from build123d import *

# Parameters (mm, degrees)
SKETCH1_R           = 31.65
BOSS_EXTRUDE1_DEPTH = 11
CUT_EXTRUDE1_DEPTH  = 35.5
SKETCH3_R           = 3.375
CUT_EXTRUDE2_DEPTH  = 21
SKETCH4_R           = 14.25
BOSS_EXTRUDE2_DEPTH = 62
SHELL1_T            = -4.2


# Read off the part's stored shape, not the designer's step: Draft1, Split1
with BuildPart() as part:
    # Sketch1 → Boss-Extrude1 (new body)
    with BuildSketch(Plane(origin=(0, 0, 0), x_dir=(1, 0, 0), z_dir=(0, 1, 0))):
        with Locations(Location((0, 0, 0), (0, 0, 270))):
            Circle(SKETCH1_R)
    extrude(amount=BOSS_EXTRUDE1_DEPTH)

    # Sketch2 → Cut-Extrude1 (cut, symmetric)
    with BuildSketch(Plane(origin=(0, 0, 0), x_dir=(0, 0, -1), z_dir=(1, 0, 0))):
        Polygon((31.65, 11), (-31.65, 4.5), (-31.65, 11), align=None)
    extrude(amount=CUT_EXTRUDE1_DEPTH, both=True, mode=Mode.SUBTRACT)

    # Sketch3 → Cut-Extrude2 (cut)
    with BuildSketch(Plane(origin=(0, 7.669134063, 0.787509817), x_dir=(1, 0, 0), z_dir=(0, 0.9947691619431022, 0.10214849214265666))):
        with Locations(Location((0, -25.899775761, 0), (0, 0, 270))):
            Circle(SKETCH3_R)
        with Locations(Location((-22.429863761, -12.94988788, 0), (0, 0, 270))):
            Circle(SKETCH3_R)
        with Locations(Location((-22.429863761, 12.94988788, 0), (0, 0, 270))):
            Circle(SKETCH3_R)
        with Locations(Location((0, 25.899775761, 0), (0, 0, 270))):
            Circle(SKETCH3_R)
        with Locations(Location((22.429863761, 12.94988788, 0), (0, 0, 270))):
            Circle(SKETCH3_R)
        with Locations(Location((22.429863761, -12.94988788, 0), (0, 0, 270))):
            Circle(SKETCH3_R)
    extrude(amount=-CUT_EXTRUDE2_DEPTH, mode=Mode.SUBTRACT)

    # Sketch4 → Boss-Extrude2 (add)
    with BuildSketch(Plane(origin=(0, 7.669134063, 0.787509817), x_dir=(1, 0, 0), z_dir=(0, 0.9947691619431022, 0.10214849214265666))):
        with Locations(Location((0, 0.791650814, 0), (0, 0, 270))):
            Circle(SKETCH4_R)
    extrude(amount=-BOSS_EXTRUDE2_DEPTH)

    # Draft1 outline → Draft1 (revolve)
    with BuildSketch(Plane(origin=(0, 0.080865937, -0.787509817), x_dir=(1, 0, 0), z_dir=(0, -0.102148492142657, 0.994769161943102))):
        Polygon((14.25, -54.290538995), (17.183507111, 1.684111168), (14.25, 1.684111168), align=None)
    revolve(axis=Axis((0, 0.080865937, -0.787509817), (0, 0.994769161943102, 0.102148492142657)))


with BuildPart() as body_2:
    # Split1: the piece on the far side of the plane
    add(part.part)
    split(bisect_by=Plane(origin=(0, 0, 0), x_dir=(1, 0, 0), z_dir=(0, 1, 0)), keep=Keep.BOTTOM)

    # Shell1
    shell1_openings = [body_2.faces().sort_by_distance(p)[0] for p in [
        (0, -53.92568804, -6.333206513),
    ]]
    offset(amount=SHELL1_T, openings=shell1_openings, kind=Kind.INTERSECTION)


with BuildPart() as part_1:
    add(part.part)

    # Split1
    split(bisect_by=Plane(origin=(0, 0, 0), x_dir=(1, 0, 0), z_dir=(0, 1, 0)), keep=Keep.TOP)


with BuildPart() as body_2_1:
    add(body_2.part)

    # Combine1: union part
    add(part_1.part)


solid = body_2_1.part
CAD build for the part. Positions are in the model's coordinates, mm. A direction names the side the tool comes from. Give positions to 0.01 mm unless a question says otherwise; leave off trailing zeros. Write each loop counter-clockwise with the first axis right and the second up, starting at its lowest first coordinate (ties: lowest second). Pieces come first, ordered by that corner, then holes. Notation, with made-up numbers: M 21.5,53 L 78.5,53 A28 ccw 78.5,83 Z; hole C -7.75,34 d6. An arc over 180 degrees is marked long. Put each result on its own line as item: value. Start each with the question number.
(1) Flat gauge pins, fed straight in: pin 1 Ø10 at (y, z) = (-18, 5) entering from -X; pin 2 Ø7.5 at (x, z) = (-4, -6) entering from -Y; pin 3 Ø3 at (x, z) = (-9, -4.5) entering from -Y. Where does each tip first touch, or does it go through?
(2) Mould opens along Y. For faces 3 (the face through (22.578, 4.717, -15.923)), 4 (the face through (-2.473, -29.177, 7.403)), 5 (the face through (0.443, 7.795, -0.443)) say: +Y half, -Y half, draft (parallel to the pull), parting line (faces both ways), or undercut.
(3) Band-saw the part on B-B, the plane z = -12. Give the number of separate pieces and of enclosed holes in the cut face, and give its area (3 significant figures).
(4) Band-saw the part on A-A, the plane x = -21. Write the cut outline in (y, z), and give its area (3 significant figures).
(5) Which spindle directions (+Z, -Z, +X, -X, +Y, -Y) get a long thin tool onto all of the face, cutting with end or side? Do faces 1 (the face through (9.699, -53.582, -9.682)), 2 (the face through (0, -4.2, -1)). Say none if no direction does.
(6) Probe L1, parallel to X at y = -32, z = -4.5; L2, parallel to Z at x = -9, y = -35; L3, parallel to X at y = -32, z = 5.5. List the from-to ranges inside material, lowest first.
(7) Band-saw the part on C-C, the plane x = 0. Write the cut outline in (y, z).
Response values:
1. pin 1: stops at x = -16.01
1. pin 2: stops at y = -4.2
1. pin 3: stops at y = -54.26
2. face 3: parting line
2. face 4: undercut
2. face 5: +Y half
3. separate pieces: 3
3. enclosed holes: 0
3. area: 1,050 mm2
4. outline: M 0,-23.68 L 10.18,-23.68 L 9.3,-15.14 L 0,-16.09 Z; M 0,-9.94 L 8.68,-9.05 L 6.66,10.63 L 0,9.94 Z; M 0,16.09 L 6.03,16.71 L 5.32,23.68 L 0,23.68 Z
4. area: 273 mm2
5. face 1: -Z, +X, -X, -Y
5. face 2: none
6. L1: x = -15.4 to -11.19, 11.19 to 15.4
6. L2: z = -16.68 to -10.76, 2.1 to 8.07
6. L3: x = -12.17 to -5.98, 5.98 to 12.17
7. outline: M -55.38,7.84 L -54.95,3.66 L -4.2,11.57 L -4.2,-13.89 L -52.9,-16.32 L -52.47,-20.51 L 0,-17.88 L 0,-22.64 L 9.97,-21.62 L 5.37,23.19 L 0,22.64 L 0,16.48 Z; M 0,-31.65 L 11,-31.65 L 10.66,-28.33 L 0,-29.43 Z; M 0,29.43 L 4.68,29.91 L 4.5,31.65 L 0,31.65 Z
